Source: three-view drawing plus pictorial views. Frame: mm from the lowest corner of the part. A direction names the side the tool comes from. Coordinates: 2 decimals unless noted, no trailing zeros. Order: outer loops, then holes, each group sorted by start corner. A loop starts at its lowest first (then second) coordinate and runs counter-clockwise, first axis right, second up. Notation, with made-up numbers: M 59.25,80 L 110.25,80 A17 ccw 110.25,94 Z; hole C 85,63.25 d8. An arc over 180 degrees is marked long. One line per question, with ' | ' between items.
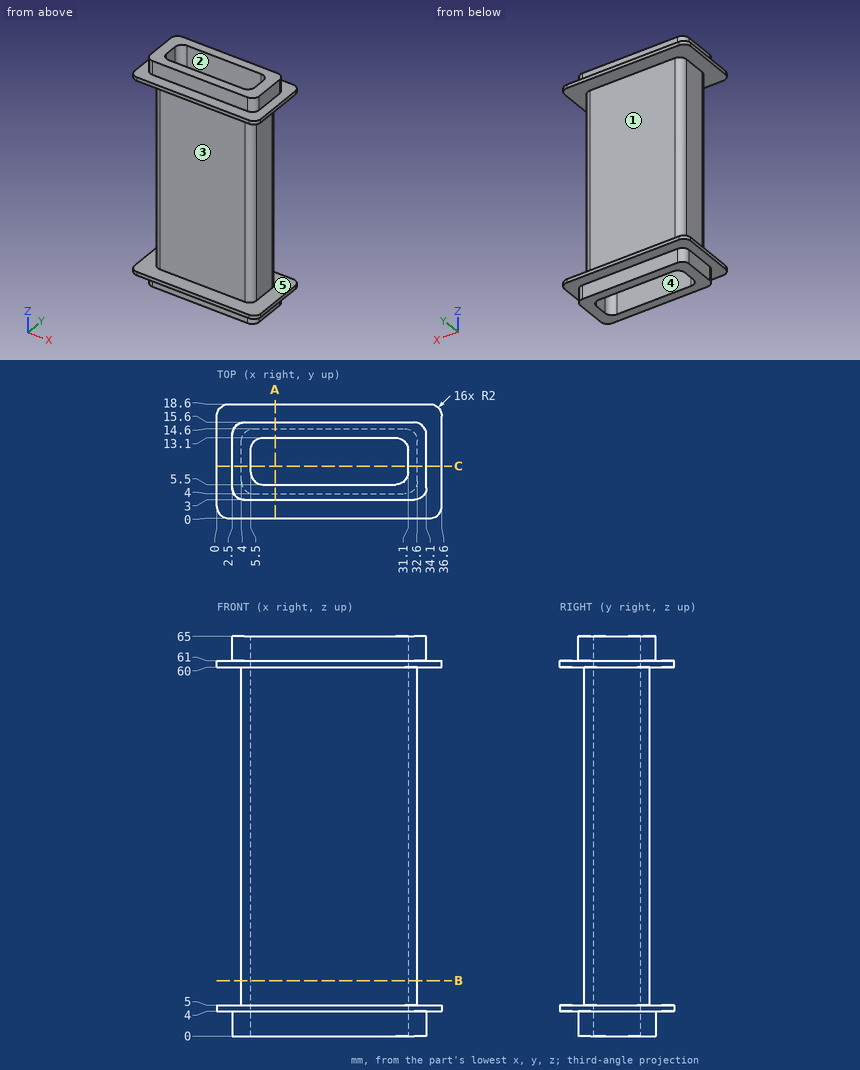
1. Material intervals for line 1 (Y direction, x = 28, z = 25); line 2 (Z direction, x = 24.5, y = 16.25); line 3 (X direction, y = 7.25, z = 26.5), sorted ascending. Write a range as [from, to].
Response values:
line 1: y = [4, 5.5], [13.1, 14.6] | line 2: z = [4, 5], [60, 61] | line 3: x = [4, 5.52], [31.08, 32.6]
2. Section A-A, the plane x = 9.5. Output: boundary loops of the cut face in (y, z).
Response values:
outline: M 0,4 L 3,4 L 3,0 L 5.5,0 L 5.5,65 L 3,65 L 3,61 L 0,61 L 0,60 L 4,60 L 4,5 L 0,5 Z; M 13.1,0 L 15.6,0 L 15.6,4 L 18.6,4 L 18.6,5 L 14.6,5 L 14.6,60 L 18.6,60 L 18.6,61 L 15.6,61 L 15.6,65 L 13.1,65 Z
3. Section B-B, the plane z = 9. Output: boundary loops of the cut face in (x, y).
Response values:
outline: M 4,6 A2 ccw 6,4 L 30.6,4 A2 ccw 32.6,6 L 32.6,12.6 A2 ccw 30.6,14.6 L 6,14.6 A2 ccw 4,12.6 Z; hole M 5.5,7.5 A2 ccw 7.5,5.5 L 29.1,5.5 A2 ccw 31.1,7.5 L 31.1,11.1 A2 ccw 29.1,13.1 L 7.5,13.1 A2 ccw 5.5,11.1 Z
4. Section C-C, the plane y = 8.5. Output: boundary loops of the cut face in (x, z), and give its area (3 significant figures).
Response values:
outline: M 0,4 L 2.5,4 L 2.5,0 L 5.5,0 L 5.5,65 L 2.5,65 L 2.5,61 L 0,61 L 0,60 L 4,60 L 4,5 L 0,5 Z; M 31.1,0 L 34.1,0 L 34.1,4 L 36.6,4 L 36.6,5 L 32.6,5 L 32.6,60 L 36.6,60 L 36.6,61 L 34.1,61 L 34.1,65 L 31.1,65 Z | area: 235 mm^2
5. Access query for the marked faces 1, 2 and 3. Directions: +Z, -Z, +X, -X, +Y, -Y. A direction counts if a zero-diameter tool reaches every point of the face in a straight line with its end or side. Return the directions, or none.
Response values:
face 1: +X, -X, +Y | face 2: +Z, -Z | face 3: +X, -X, -Y
6. Draft query along Z for the marked faces 4 and 5. Return one class per face: pulls with the +Z half, pulls with the -Z half, needs draft (parallel to the pull), parting line crosses it, or undercut.
Response values:
face 4: needs draft | face 5: undercut
7. Pin query (flat end, axial travel): P1, Ø10, axis at x = 29.5, z = 43, coming from the -Y side; P2, Ø1.2, axis at y = 7, z = 1, coming from the +X side; P3, Ø9.5, axis at x = 16.5, y = 12, coming from the +Z side; P4, Ø3, axis at y = 9, z = 9, coming from the -X side. Return the tip coordinate at first contact, or that it passes through.
Response values:
P1: stops at y = 4 | P2: stops at x = 34.1 | P3: stops at z = 65 | P4: stops at x = 4
